Design review of the part built by this model. Coordinates are the model's own, in mm. Face numbers are marked on the shaded views. A direction names the side the tool comes from. Give positions to 0.01 mm unless a question says otherwise; leave off trailing zeros. Loops run counter-clockwise (first coordinate to the right, second up) from the corner with the lowest first, then second, coordinate; pieces in that order, holes last. Notation, with made-up numbers: (62, 8.25) - (106, 8.25) arc R12 cw to (106, 28.25) - close; hole circle Ø10 at (74, 1). An arc over 180 degrees is marked (long way). Write each question's results on one line, items separated by ' | '.
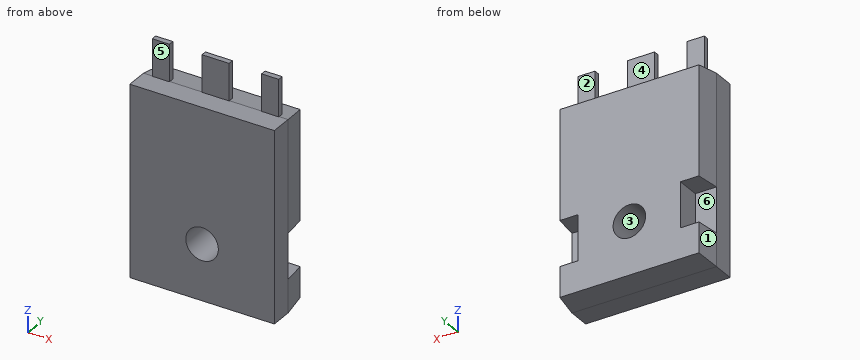
from build123d import *
from OCP.BRepFilletAPI import BRepFilletAPI_MakeChamfer

# Parameters (mm, degrees)
SKETCH1_W           = 16
SKETCH1_H           = 21
BOSS_EXTRUDE1_DEPTH = 5
SKETCH2_W           = 2.338235294
SKETCH2_H           = 5
CUT_EXTRUDE1_DEPTH  = 2.6
SKETCH3_R           = 1.8
CUT_EXTRUDE2_DEPTH  = 15.115594213
CHAMFER1_SIZE       = 2.6
CHAMFER1_SIZE2      = 0.3
SKETCH4_W           = 1.9
SKETCH4_H           = 0.6
SKETCH4_W_2         = 3
BOSS_EXTRUDE2_DEPTH = 4.5
SKETCH5_W           = 1.2
SKETCH5_H           = 0.6
BOSS_EXTRUDE3_DEPTH = 15.5
CHAMFER2_SIZE       = 0.4
CHAMFER3_SIZE       = 1
CHAMFER4_SIZE       = 0.5
SKETCH6_W           = 21.119407152
SKETCH6_H           = 13.185156935
CUT_EXTRUDE3_DEPTH  = 32.669425318
SKETCH7_W           = 15.715970721
SKETCH7_H           = 3.676449557
CUT_EXTRUDE4_DEPTH  = 20.696256624


with BuildPart() as part:
    # Sketch1 → Boss-Extrude1 (new body)
    with BuildSketch(Plane(origin=(0, 0, 0), x_dir=(1, 0, 0), z_dir=(0, 1, 0))):
        Rectangle(SKETCH1_W, SKETCH1_H)
    extrude(amount=BOSS_EXTRUDE1_DEPTH)

    # Sketch2 → Cut-Extrude1 (cut)
    with BuildSketch(Plane(origin=(0, 5, 0), x_dir=(1, 0, 0), z_dir=(0, 1, 0))):
        with Locations((-6.830882353, 4.35)):
            Rectangle(SKETCH2_W, SKETCH2_H)
        with Locations((6.830882353, 4.35)):
            Rectangle(SKETCH2_W, SKETCH2_H)
    extrude(amount=-CUT_EXTRUDE1_DEPTH, mode=Mode.SUBTRACT)

    # Sketch3 → Cut-Extrude2 (cut, through all)
    with BuildSketch(Plane(origin=(0, 5, 0), x_dir=(1, 0, 0), z_dir=(0, 1, 0))):
        with Locations(Location((0, 4.35, 0), (0, 0, 270))):
            Circle(SKETCH3_R)
    extrude(amount=-CUT_EXTRUDE2_DEPTH, mode=Mode.SUBTRACT)

    # Chamfer1: one chamfer whose edges measure the first distance from different faces: ONE call of the kernel's chamfer builder (chamfer() names one face for all edges)
    chamfer1_edges_1 = [part.edges().sort_by_distance(p)[0] for p in [
        (8, 5, 4.325),
        (8, 5, -8.675),
    ]]
    chamfer1_side_1 = [part.faces().sort_by_distance(p)[0] for p in [
        (8, 2.330434783, 0.614673913),
    ]]
    chamfer1_edges_2 = [part.edges().sort_by_distance(p)[0] for p in [
        (-8, 5, 4.325),
        (-8, 5, -8.675),
    ]]
    chamfer1_side_2 = [part.faces().sort_by_distance(p)[0] for p in [
        (-8, 2.330434783, 0.614673913),
    ]]
    chamfer1_edges_3 = [part.edges().sort_by_distance(p)[0] for p in [
        (0, 5, -10.5),
    ]]
    chamfer1_side_3 = [part.faces().sort_by_distance(p)[0] for p in [
        (0, 2.5, -10.5),
    ]]
    chamfer1_edges_4 = [part.edges().sort_by_distance(p)[0] for p in [
        (0, 5, 10.5),
    ]]
    chamfer1_side_4 = [part.faces().sort_by_distance(p)[0] for p in [
        (0, 2.5, 10.5),
    ]]
    chamfer1 = BRepFilletAPI_MakeChamfer(part.part.solid().wrapped)
    for e in chamfer1_edges_1:
        chamfer1.Add(CHAMFER1_SIZE, CHAMFER1_SIZE2, e.wrapped, chamfer1_side_1[0].wrapped)  # the first distance lies on this face
    for e in chamfer1_edges_2:
        chamfer1.Add(CHAMFER1_SIZE, CHAMFER1_SIZE2, e.wrapped, chamfer1_side_2[0].wrapped)  # the first distance lies on this face
    for e in chamfer1_edges_3:
        chamfer1.Add(CHAMFER1_SIZE, CHAMFER1_SIZE2, e.wrapped, chamfer1_side_3[0].wrapped)  # the first distance lies on this face
    for e in chamfer1_edges_4:
        chamfer1.Add(CHAMFER1_SIZE, CHAMFER1_SIZE2, e.wrapped, chamfer1_side_4[0].wrapped)  # the first distance lies on this face
    add(Compound.cast(chamfer1.Shape()), mode=Mode.REPLACE)

    # Sketch4 → Boss-Extrude2 (add)
    with BuildSketch(Plane.XY.offset(10.5)):
        with Locations((-6.05, 2.65)):
            Rectangle(SKETCH4_W, SKETCH4_H)
        with Locations((6.05, 2.65)):
            Rectangle(SKETCH4_W, SKETCH4_H)
        with Locations((0, 2.65)):
            Rectangle(SKETCH4_W_2, SKETCH4_H)
    extrude(amount=BOSS_EXTRUDE2_DEPTH)

    # Sketch5 → Boss-Extrude3 (add)
    with BuildSketch(Plane.XY.offset(15)):
        with Locations((-6.05, 2.65)):
            Rectangle(SKETCH5_W, SKETCH5_H)
        with Locations((0, 2.65)):
            Rectangle(SKETCH5_W, SKETCH5_H)
        with Locations((6.05, 2.65)):
            Rectangle(SKETCH5_W, SKETCH5_H)
    extrude(amount=BOSS_EXTRUDE3_DEPTH)

    # Chamfer2
    # the kernel refuses this chamfer: 0.4 mm, written as the material it adds along each edge
    with BuildSketch(Plane(origin=(-5.45, 2.35, 15), x_dir=(0.9996219169112966, 0, -0.027495876610587302), z_dir=(0, 1, 0))) as chamfer2_piece_1_section:
        Polygon((CHAMFER2_SIZE * 0.999621916911, -CHAMFER2_SIZE * 0.0274958766106), (-CHAMFER2_SIZE * 0.0274958766106, -CHAMFER2_SIZE * 0.999621916911), (0, 0), align=None)
    chamfer2_piece_1 = extrude(amount=0.6, mode=Mode.PRIVATE)
    chamfer2_piece_1 = split(chamfer2_piece_1, bisect_by=Plane(origin=(-5.1, 2.65, 15.135195933), z_dir=(-1, 0, 0)), keep=Keep.TOP, mode=Mode.PRIVATE)
    add(chamfer2_piece_1)
    with BuildSketch(Plane(origin=(6.65, 2.95, 15), x_dir=(0.9996219169112966, 0, -0.027495876610587302), z_dir=(0, -1, 0))) as chamfer2_piece_2_section:
        Polygon((CHAMFER2_SIZE * 0.999621916911, CHAMFER2_SIZE * 0.0274958766106), (-CHAMFER2_SIZE * 0.0274958766106, CHAMFER2_SIZE * 0.999621916911), (0, 0), align=None)
    chamfer2_piece_2 = extrude(amount=0.6, mode=Mode.PRIVATE)
    chamfer2_piece_2 = split(chamfer2_piece_2, bisect_by=Plane(origin=(7, 2.65, 15.135195933), z_dir=(-1, 0, 0)), keep=Keep.TOP, mode=Mode.PRIVATE)
    add(chamfer2_piece_2)
    with BuildSketch(Plane(origin=(5.45, 2.35, 15), x_dir=(-0.9996219169112966, 0, -0.027495876610587302), z_dir=(0, 1, 0))) as chamfer2_piece_3_section:
        Polygon((CHAMFER2_SIZE * 0.999621916911, CHAMFER2_SIZE * 0.0274958766106), (-CHAMFER2_SIZE * 0.0274958766106, CHAMFER2_SIZE * 0.999621916911), (0, 0), align=None)
    chamfer2_piece_3 = extrude(amount=0.6, mode=Mode.PRIVATE)
    chamfer2_piece_3 = split(chamfer2_piece_3, bisect_by=Plane(origin=(5.1, 2.65, 15.135195933), z_dir=(1, 0, 0)), keep=Keep.TOP, mode=Mode.PRIVATE)
    add(chamfer2_piece_3)
    with BuildSketch(Plane(origin=(-6.65, 2.95, 15), x_dir=(-0.9996219169112966, 0, -0.027495876610587302), z_dir=(0, -1, 0))) as chamfer2_piece_4_section:
        Polygon((CHAMFER2_SIZE * 0.999621916911, -CHAMFER2_SIZE * 0.0274958766106), (-CHAMFER2_SIZE * 0.0274958766106, -CHAMFER2_SIZE * 0.999621916911), (0, 0), align=None)
    chamfer2_piece_4 = extrude(amount=0.6, mode=Mode.PRIVATE)
    chamfer2_piece_4 = split(chamfer2_piece_4, bisect_by=Plane(origin=(-7, 2.65, 15.135195933), z_dir=(1, 0, 0)), keep=Keep.TOP, mode=Mode.PRIVATE)
    add(chamfer2_piece_4)

    # Chamfer3
    # the kernel refuses this chamfer: 1 mm, written as the material it adds along each edge
    with BuildSketch(Plane(origin=(0.6, 2.35, 15), x_dir=(0.9996219169112968, 0, -0.027495876610585623), z_dir=(0, 1, 0))) as chamfer3_piece_1_section:
        Polygon((CHAMFER3_SIZE * 0.999621916911, -CHAMFER3_SIZE * 0.0274958766106), (-CHAMFER3_SIZE * 0.0274958766106, -CHAMFER3_SIZE * 0.999621916911), (0, 0), align=None)
    chamfer3_piece_1 = extrude(amount=0.6, mode=Mode.PRIVATE)
    chamfer3_piece_1 = split(chamfer3_piece_1, bisect_by=Plane(origin=(1.5, 2.65, 15.335900747), z_dir=(-1, 0, 0)), keep=Keep.TOP, mode=Mode.PRIVATE)
    add(chamfer3_piece_1)
    with BuildSketch(Plane(origin=(-0.6, 2.95, 15), x_dir=(0.02749587661058645, 0, 0.9996219169112968), z_dir=(0, -1, 0))) as chamfer3_piece_2_section:
        Polygon((CHAMFER3_SIZE * 0.999621916911, CHAMFER3_SIZE * 0.0274958766106), (-CHAMFER3_SIZE * 0.0274958766106, CHAMFER3_SIZE * 0.999621916911), (0, 0), align=None)
    chamfer3_piece_2 = extrude(amount=0.6, mode=Mode.PRIVATE)
    chamfer3_piece_2 = split(chamfer3_piece_2, bisect_by=Plane(origin=(-1.5, 2.65, 15.335900747), z_dir=(1, 0, 0)), keep=Keep.TOP, mode=Mode.PRIVATE)
    add(chamfer3_piece_2)

    # Chamfer4
    chamfer4_edges = [part.edges().sort_by_distance(p)[0] for p in [
        (5.45, 2.65, 30.5),
        (6.65, 2.65, 30.5),
        (0.6, 2.65, 30.5),
        (-0.6, 2.65, 30.5),
        (-5.45, 2.65, 30.5),
        (-6.65, 2.65, 30.5),
    ]]
    chamfer(chamfer4_edges, length=CHAMFER4_SIZE)

    # Sketch6 → Cut-Extrude3 (cut, through all)
    with BuildSketch(Plane(origin=(0, 2.95, 0), x_dir=(1, 0, 0), z_dir=(0, 1, 0))):
        with Locations((0.165735258, -24.347578467)):
            Rectangle(SKETCH6_W, SKETCH6_H)
    extrude(amount=-CUT_EXTRUDE3_DEPTH, mode=Mode.SUBTRACT)

    # Sketch7 → Cut-Extrude4 (cut, through all)
    with BuildSketch(Plane(origin=(0, 2.95, 0), x_dir=(1, 0, 0), z_dir=(0, 1, 0))):
        with Locations((-0.142014639, -16.413224779)):
            Rectangle(SKETCH7_W, SKETCH7_H)
    extrude(amount=-CUT_EXTRUDE4_DEPTH, mode=Mode.SUBTRACT)


solid = part.part
(1) Draft analysis for pull direction X (two halves, no side actions). For the marked faces 1, 2 and 3, state which applies: pulls with the +X half, pulls with the -X half, needs draft (parallel to the pull), parting line crosses it, or undercut.
Answers below:
face 1: pulls with the -X half | face 2: needs draft | face 3: undercut
(2) Insertion check: P1, Ø1.5, axis at x = -6.5, z = 12.5, coming from the +Y side; P2, Ø1.2, axis at x = -7, y = 4, coming from the +Z side; P3, Ø0.5, axis at y = 2.5, z = 12, coming from the -X side. Each pin has a flat end and moves straight along its axis. Give the tip position at first contact, or say it passes through.
Answers below:
P1: y = 2.95 | P2: z = 10.38 | P3: x = -7
(3) Take a section at A-A on z = -4.35. Give the boundary of the cut face in (x, y).
Answers below:
outline: (-8, 0) - (-1.8, 0) - (-1.8, 5) - (-5.66, 5) - (-5.66, 2.4) - (-8, 2.4) - close; (1.8, 0) - (8, 0) - (8, 2.4) - (5.66, 2.4) - (5.66, 5) - (1.8, 5) - close
(4) Take a section at B-B on x = 0. Give the boundary of the cut face in (y, z) (3 decimals).
Answers below:
outline: (0, -10.5) - (2.4, -10.5) - (5, -10.2) - (5, -6.15) - (0, -6.15) - close; (0, -2.55) - (5, -2.55) - (5, 10.2) - (2.4, 10.5) - (2.95, 10.5) - (2.95, 14.575) - (2.35, 14.575) - (2.35, 10.5) - (0, 10.5) - close
(5) Tool access review of the marked faces 4, 5 and 6: name each direction out of +Z, -Z, +X, -X, +Y, -Y from which nothing blocks a thin tool from reaching the whole face with its end or side.
Answers below:
face 4: +Z, +X, -X, +Y | face 5: +Z, +X, -X, -Y | face 6: -X, +Y
(6) Take a section at D-D on x = 7.25. Give the boundary of the cut face in (y, z), plus the area to 3 significant figures.
Answers below:
outline: (0, -10.5) - (2.4, -10.5) - (5, -10.2) - (5, -6.85) - (2.4, -6.85) - (2.4, -1.85) - (5, -1.85) - (5, 10.2) - (2.4, 10.5) - (0, 10.5) - close | area: 91.2 mm2
(7) Take a section at C-C on y = 1.4. Give the boundary of the cut face in (x, z), plus the area to 3 significant figures.
Answers below:
outline: (-8, -10.5) - (8, -10.5) - (8, 10.5) - (-8, 10.5) - close; hole circle Ø3.6 at (0, -4.35) | area: 326 mm2
(8) Wall thickness on line 1 along X through (y, z) = (2.9, 11.75); line 2 along X through (y, z) = (3.9, -4.35); line 3 along X through (y, z) = (1.75, -4.35): over which ranges is each line inside the solid? List them lowest first. Write a range as from..to.
Answers below:
line 1: -7..-5.1, -1.5..1.5, 5.1..7 | line 2: -5.66..-1.8, 1.8..5.66 | line 3: -8..-1.8, 1.8..8
